Read the model definition and answer for the solid it produces. Units are mm, in the model's axes. Face numbers are marked on the shaded views. Round coordinates to 2 decimals unless told otherwise and drop trailing zeros. Order: outer loops, then holes, each group sorted by start corner. A loop starts at its lowest first (then second) coordinate and runs counter-clockwise, first axis right, second up. Notation, with made-up numbers: (87.25, 13) - (97.25, 13) arc R11 cw to (97.25, 19) - close; hole circle Ø5 at (8.5, 16.5). An arc over 180 degrees is marked (long way). Put each result on its own line as item: value. Start each with the question number.
Q1. Section B-B on z = 18 is taken. Give the vertices of the cut face in (x, y), then the cut area to 3 significant figures.
Q2. This flat-tipped pin is pushed along its axis until it touches: pin 1 Ø8 at (x, z) = (-10.5, 38) entering from -Y. Where does it stop, or does it pass through?
Q3. For a pull along X with two mould halves and no side action, classify the marked faces 1, 2, 3 and 4 as pulls with the +X half, pulls with the -X half, needs draft (parallel to the pull), parting line crosses it, or undercut.
Q4. Section A-A on y = -29 is taken. Give the vertices of the cut face in (x, z).
Q5. Find the intervals of material crossed by line 1 along X through (y, z) = (-28.5, 6); line 2 along Y through (x, z) = (17.5, 29), in increasing order. Write a range as from..to.
Q6. Section C-C on x = -4.5 is taken. Give the vertices of the cut face in (y, z), then the cut area to 3 significant figures.
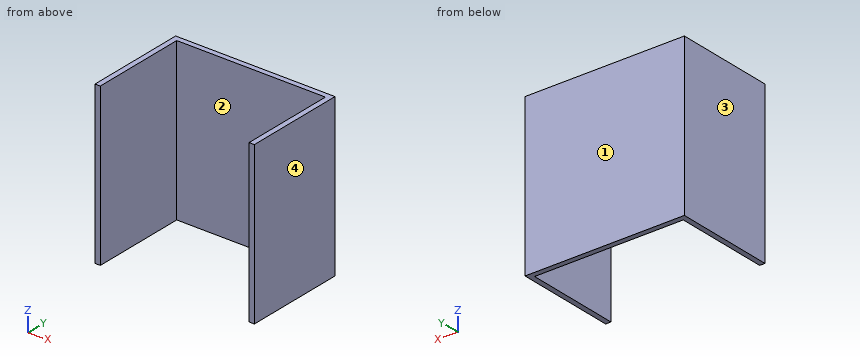
from build123d import *

# Parameters (mm, degrees)
SKETCH1_W           = 60
SKETCH1_H           = 60
BOSS_EXTRUDE1_DEPTH = 2
SKETCH2_W           = 2
SKETCH2_H           = 60
BOSS_EXTRUDE2_DEPTH = 36


with BuildPart() as part:
    # Sketch1 → Boss-Extrude1 (new body)
    with BuildSketch(Plane(origin=(0, 0, 0), x_dir=(1, 0, 0), z_dir=(0, 1, 0))):
        with Locations((4.971289332, -16.330275229)):
            Rectangle(SKETCH1_W, SKETCH1_H)
    extrude(amount=BOSS_EXTRUDE1_DEPTH)

    # Sketch2 → Boss-Extrude2 (add)
    with BuildSketch(Plane.XZ):
        with Locations((33.971289332, 16.330275229)):
            Rectangle(SKETCH2_W, SKETCH2_H)
        with Locations((-24.028710668, 16.330275229)):
            Rectangle(SKETCH2_W, SKETCH2_H)
    extrude(amount=BOSS_EXTRUDE2_DEPTH)


solid = part.part
Findings:
1. outline: (-25.03, -36) - (-23.03, -36) - (-23.03, 0) - (32.97, 0) - (32.97, -36) - (34.97, -36) - (34.97, 2) - (-25.03, 2) - close
1. area: 264 mm2
2. pin 1: y = 0
3. face 1: needs draft
3. face 2: undercut
3. face 3: pulls with the -X half
3. face 4: pulls with the +X half
4. outline: (-25.03, -13.67) - (-23.03, -13.67) - (-23.03, 46.33) - (-25.03, 46.33) - close; (32.97, -13.67) - (34.97, -13.67) - (34.97, 46.33) - (32.97, 46.33) - close
5. line 1: -25.03..-23.03, 32.97..34.97
5. line 2: 0..2
6. outline: (0, -13.67) - (2, -13.67) - (2, 46.33) - (0, 46.33) - close
6. area: 120 mm2
